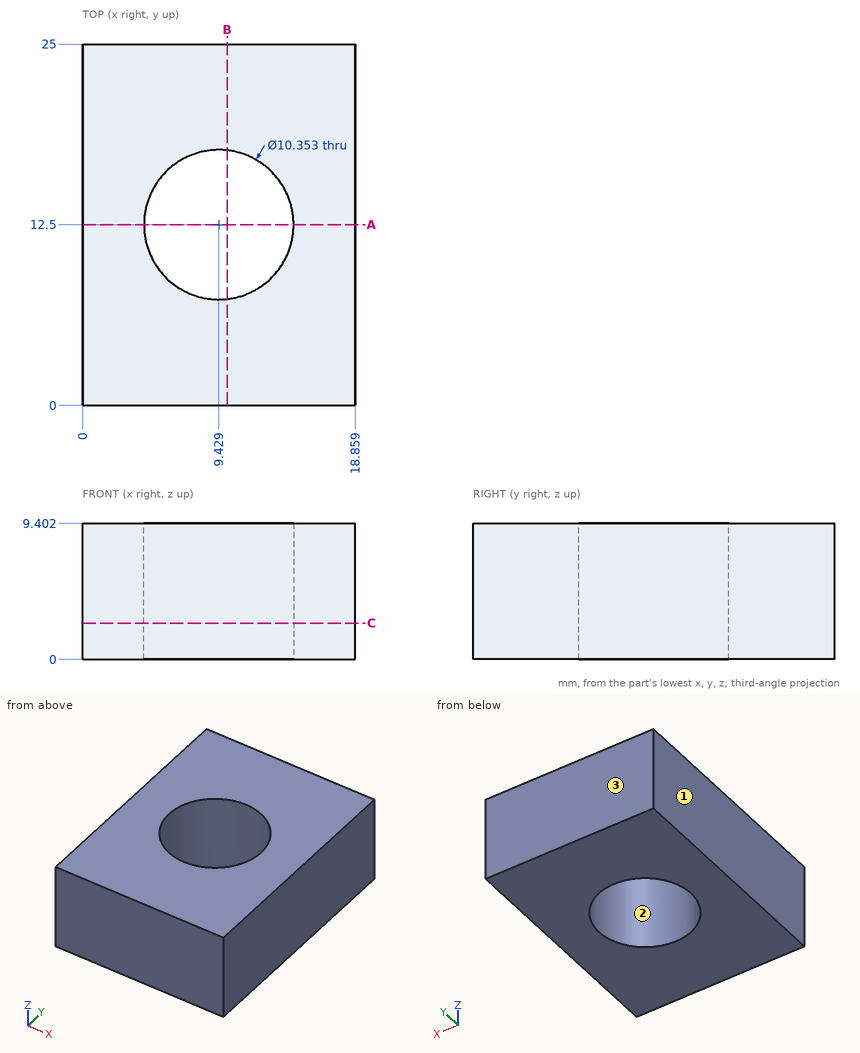
Here's the drawing with two shaded views (mm, measured from the low corner). I have some questions. Give positions to 0.01 mm unless a question says otherwise; leave off trailing zeros. Write each loop counter-clockwise with the first axis right and the second up, starting at its lowest first coordinate (ties: lowest second). Pieces come first, ordered by that corner, then holes. Notation, with made-up numbers: (19, 37.25) -> (43, 37.25) arc R23 cw to (43, 47.25) -> close; hole circle Ø7 at (81.5, 65). An arc over 180 degrees is marked (long way). Answer as a JSON object with one key per item and string values. Group by question number.
Item 1: Suppose I cut it at C-C (z = 2.5). Please give me the cut outline in (x, y).
Item 2: We'd pull the mould along X, two halves only. Please class the marked faces 1, 2 and 3: +X half, -X half, draft (parallel to the pull), parting line (faces both ways), or undercut.
Item 3: Suppose I cut it at A-A (y = 12.5). Please give me the cut outline in (x, z).
Item 4: Suppose I cut it at B-B (x = 10). Please give me the cut outline in (y, z) (1 decimal), plus the area to 3 significant figures.
Item 5: Please list where these lines run through material, in increasing order: line 1 (X direction, y = 12.25, z = 6.5); line 2 (X direction, y = 14.5, z = 6.5) (1 decimal); line 3 (Y direction, x = 13.25, z = 3.5) (1 decimal). Write a range as [from, to].
Item 6: I'm going to push a flat-ended pin straight in: P1, Ø5, axis at x = 9, y = 10, coming from the +Z side. Where does the tip first touch, or does it pass through?
Findings:
{
 "1": {"outline": "(0, 0) -> (18.86, 0) -> (18.86, 25) -> (0, 25) -> close; hole circle Ø10.35 at (9.43, 12.5)"},
 "2": {"face 1": "-X half", "face 2": "undercut", "face 3": "draft"},
 "3": {"outline": "(0, 0) -> (4.25, 0) -> (4.25, 9.4) -> (0, 9.4) -> close; (14.61, 0) -> (18.86, 0) -> (18.86, 9.4) -> (14.61, 9.4) -> close"},
 "4": {"outline": "(0, 0) -> (7.4, 0) -> (7.4, 9.4) -> (0, 9.4) -> close; (17.6, 0) -> (25, 0) -> (25, 9.4) -> (17.6, 9.4) -> close", "area": "138 mm²"},
 "5": {"line 1": "x = [0, 4.26], [14.6, 18.86]", "line 2": "x = [0, 4.7], [14.2, 18.9]", "line 3": "y = [0, 9], [16, 25]"},
 "6": {"P1": "passes through"}
}
